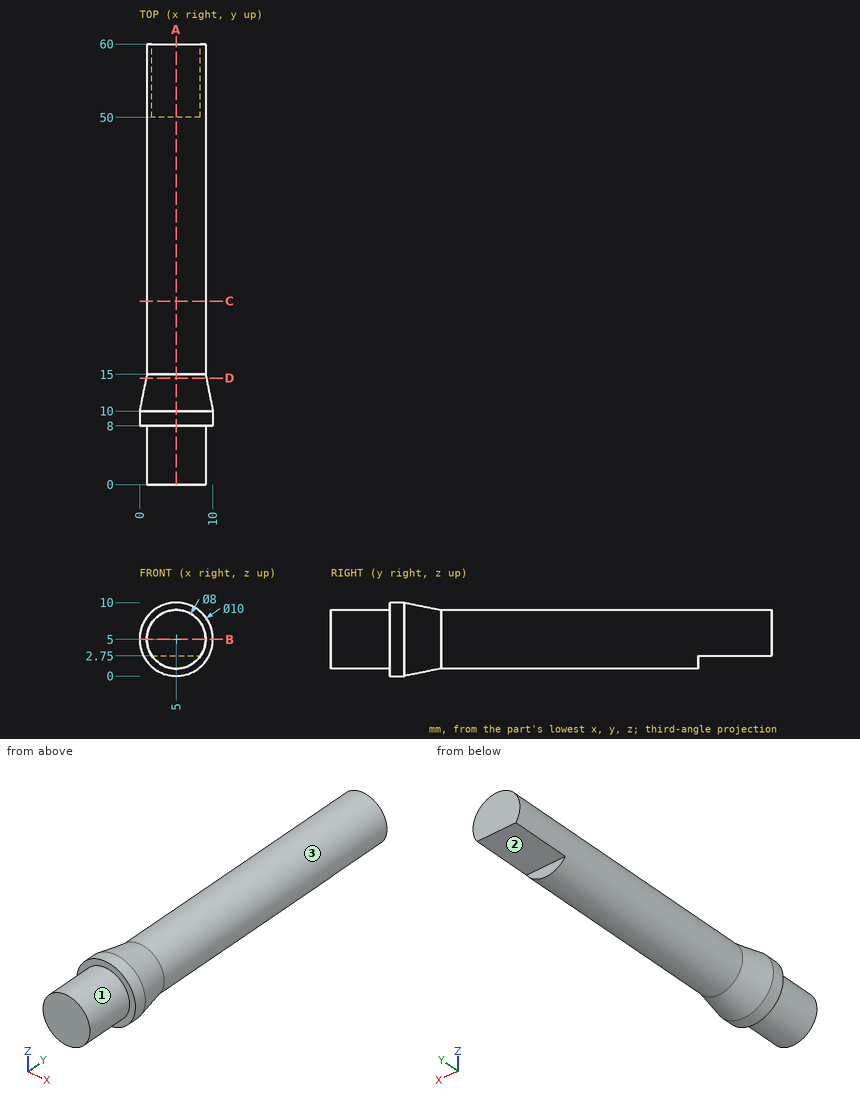
Part print with two shaded views. Sizes in mm from the minimum x, y, z corner. A direction names the side the tool comes from. Give positions to 0.01 mm unless a question says otherwise; leave off trailing zeros. Order: outer loops, then holes, each group sorted by start corner. A loop starts at its lowest first (then second) coordinate and runs counter-clockwise, first axis right, second up. Notation, with made-up numbers: M 63.5,13.25 L 118.5,13.25 A24 cw 118.5,49.25 Z; hole C 89,14.25 d5. An arc over 180 degrees is marked long. Write item = value, one per line.
Q1. Cut at A-A, the plane x = 5. List the corners of the cut face in (y, z), then the cut area to 4 significant figures.
Derived:
outline = M 0,1 L 8,1 L 8,0 L 10,0 L 15,1 L 50,1 L 50,2.75 L 60,2.75 L 60,9 L 15,9 L 10,10 L 8,10 L 8,9 L 0,9 Z
area = 471.5 mm2
Q2. Flat gauge pins, fed straight in: pin 1 (1 mm diameter, centred on x = 5, y = 38.5, fed in from -Z); pin 2 (3 mm diameter, centred on y = 53.5, z = 4.5, fed in from -X); pin 3 (6 mm diameter, centred on x = 8, z = 2.5, fed in from -Y); pin 4 (2 mm diameter, centred on y = 45.5, z = 1.5, fed in from +X). Where does each tip first touch, or does it go through?
Derived:
pin_1 = 1
pin_2 = 1
pin_3 = 0
pin_4 = 8.12
Q3. Cut at C-C, the plane y = 25. List the corners of the cut face in (x, z).
Derived:
outline = C 5,5 d8
Q4. Cut at D-D, the plane y = 14.5. List the corners of the cut face in (x, z), then the cut area to 3 significant figures.
Derived:
outline = C 5,5 d8.2
area = 52.8 mm2
Q5. Cut at B-B, the plane z = 5. List the corners of the cut face in (x, y), then the cut area to 3 significant figures.
Derived:
outline = M 0,8 L 1,8 L 1,0 L 9,0 L 9,8 L 10,8 L 10,10 L 9,15 L 9,60 L 1,60 L 1,15 L 0,10 Z
area = 489 mm2
Q6. Drill centre lines: line 1 (Y direction, x = 3.5, z = 1.5); line 2 (X direction, y = 46, z = 5); line 3 (Z direction, x = 2.5, y = 13). Where is each one in solid material? Low to high. Write a range as [from, to].
Derived:
line_1 = [0, 50]
line_2 = [1, 9]
line_3 = [1.38, 8.62]
Q7. Tool access for the marked faces 1, 2 and 3: list every direction of +Z, -Z, +X, -X, +Y, -Y with a clear straight run to the whole face (end or side of a thin tool).
Derived:
face_1 = -Y
face_2 = -Z, +X, -X, +Y
face_3 = +Y
